from build123d import *

# Parameters (mm, degrees)
SKETCH1_W                        = 18.796
SKETCH1_H                        = 18.796
SKETCH1_W_2                      = 17.272
SKETCH1_H_2                      = 17.272
BOSS_EXTRUDE1_DEPTH              = 76.2
SKETCH2_W                        = 18.796
SKETCH2_H                        = 18.796
BOSS_EXTRUDE2_DEPTH              = 2.032
F_10_0_1935_DIAMETER_HOLE1_D     = 4.572
F_10_0_1935_DIAMETER_HOLE1_DEPTH = 6.35
F_10_0_1935_DIAMETER_HOLE1_TIP   = 1.373567375


with BuildPart() as part:
    # Sketch1 → Boss-Extrude1 (new body)
    with BuildSketch(Plane(origin=(0, 0, 0), x_dir=(1, 0, 0), z_dir=(0, 1, 0))):
        Rectangle(SKETCH1_W, SKETCH1_H)
        Rectangle(SKETCH1_W_2, SKETCH1_H_2, mode=Mode.SUBTRACT)
    extrude(amount=BOSS_EXTRUDE1_DEPTH)

    # Sketch2 → Boss-Extrude2 (add)
    with BuildSketch(Plane.XZ):
        Rectangle(SKETCH2_W, SKETCH2_H)
    extrude(amount=BOSS_EXTRUDE2_DEPTH)

    # #10 (0.1935) Diameter Hole1
    with Locations(Plane(origin=(0, -2.032, 0), x_dir=(-1, 0, 0), z_dir=(0, -1, 0))):
        with Locations((0, 0)):
            Hole(F_10_0_1935_DIAMETER_HOLE1_D / 2, depth=F_10_0_1935_DIAMETER_HOLE1_DEPTH)
            with Locations((0, 0, -(F_10_0_1935_DIAMETER_HOLE1_DEPTH + F_10_0_1935_DIAMETER_HOLE1_TIP / 2))):  # 118° drill point
                Cone(0, F_10_0_1935_DIAMETER_HOLE1_D / 2, F_10_0_1935_DIAMETER_HOLE1_TIP, mode=Mode.SUBTRACT)


solid = part.part
Work out the finished part from the listing and answer in its coordinate system (mm). A direction names the side the tool comes from. Give positions to 0.01 mm unless a question says otherwise; leave off trailing zeros. Order: outer loops, then holes, each group sorted by start corner. A loop starts at its lowest first (then second) coordinate and runs counter-clockwise, first axis right, second up. Notation, with made-up numbers: (62, 61.25) - (119, 61.25) arc R25 ccw to (119, 100.25) - close; hole circle Ø10 at (-30, 13.25). An arc over 180 degrees is marked (long way). Answer as CSV lines item,"result". Start each with the question number.
Q1. The part is cut by section C-C (z = 0). Write down the section's boundary in (x, y).
Q2. Given pin 1 Ø5 at (x, z) = (-4, -2.5) entering from +Y, flat-ended and moving along its own axis, determine where the tip first touches the part or whether it passes through.
Q3. The part is cut by section D-D (z = 5.75). Write down the section's boundary in (x, y), then the cut area to 3 significant figures.
Q4. The part is cut by section A-A (x = 0). Write down the section's boundary in (y, z), then the cut area to 3 significant figures.
Q5. The mould has two halves that part along X. Classify faces 1 (the face through (0, 38, 8.636)), 2 (the face through (9.398, 38, 0)), 3 (the face through (-1, 76.2, 9)): +X half, -X half, draft (parallel to the pull), parting line (faces both ways), or undercut.
Q6. For faces 4 (the face through (0, 38, -9.398)), 5 (the face through (2, 0, 2)), determine the directions among +Z, -Z, +X, -X, +Y, -Y from which every point of the face is accessible in a straight line to the end or side of a thin tool.
Q7. Find the intervals of material crossed by L1, parallel to Z at x = -5, y = 67.5; L2, parallel to Z at x = 0, y = -0.4, in increasing order. Write a range as [from, to].
Q8. The part is cut by section B-B (y = 58). Write down the section's boundary in (x, z), then the cut area to 3 significant figures.
Check result:
1,outline,"(-9.4, -2.03) - (-2.29, -2.03) - (-2.29, 0) - (-8.64, 0) - (-8.64, 76.2) - (-9.4, 76.2) - close; (2.29, -2.03) - (9.4, -2.03) - (9.4, 76.2) - (8.64, 76.2) - (8.64, 0) - (2.29, 0) - close"
2,pin 1,"stops at y = 0"
3,outline,"(-9.4, -2.03) - (9.4, -2.03) - (9.4, 76.2) - (8.64, 76.2) - (8.64, 0) - (-8.64, 0) - (-8.64, 76.2) - (-9.4, 76.2) - close"
3,area,"154 mm²"
4,outline,"(-2.03, -9.4) - (76.2, -9.4) - (76.2, -8.64) - (0, -8.64) - (0, -2.29) - (-2.03, -2.29) - close; (-2.03, 2.29) - (0, 2.29) - (0, 8.64) - (76.2, 8.64) - (76.2, 9.4) - (-2.03, 9.4) - close"
4,area,"145 mm²"
5,face 1,"undercut"
5,face 2,"+X half"
5,face 3,"draft"
6,face 4,"-Z, +X, -X, +Y, -Y"
6,face 5,"+Y"
7,L1,"z = [-9.4, -8.64], [8.64, 9.4]"
7,L2,"z = [-9.4, -2.29], [2.29, 9.4]"
8,outline,"(-9.4, -9.4) - (9.4, -9.4) - (9.4, 9.4) - (-9.4, 9.4) - close; hole (-8.64, -8.64) - (8.64, -8.64) - (8.64, 8.64) - (-8.64, 8.64) - close"
8,area,"55.0 mm²"
